```python
from build123d import *

# Parameters (mm, degrees)
F1_DEPTH = 2
F2_R     = 4.445875
F3_DEPTH = 6
F4_R     = 4.445875
F5_DEPTH = 3
F6_R     = 1.6
F7_DEPTH = 11.001


with BuildPart() as f1:
    # F0 (on Top) → F1 (new body)
    with BuildSketch(Plane.XY):
        Polygon((20, 9.5026303193), (0, 18.5309549122), (-20, 9.5026303193), (-20, -12.4407204949), (0, -21.4690450878), (20, -12.4407204949), align=None)
    extrude(amount=-F1_DEPTH)

    # F2 (on face) → F3 (join)
    with BuildSketch(Plane.XY):
        Circle(F2_R)
    extrude(amount=F3_DEPTH)

    # F4 (on face) → F5 (join)
    with BuildSketch(Plane(origin=(0, 0, -2), x_dir=(1, 0, 0), z_dir=(0, 0, -1))):
        Circle(F4_R)
    extrude(amount=F5_DEPTH)

    # F6 (on face) → F7 (cut, through all)
    with BuildSketch(Plane.XY.offset(6)):
        Circle(F6_R)
    extrude(amount=-F7_DEPTH, mode=Mode.SUBTRACT)


solid = f1.part
```
Geometry: final body of the model. Coordinates: model frame, mm. A direction names the side the tool comes from. Coordinates: 2 decimals unless noted, no trailing zeros. Order: outer loops, then holes, each group sorted by start corner. A loop starts at its lowest first (then second) coordinate and runs counter-clockwise, first axis right, second up. Notation, with made-up numbers: M 17,24.5 L 38,24.5 A26 cw 38,46.5 Z; hole C -33,28.5 d11. An arc over 180 degrees is marked long. Answer in a Markdown table with one row per item. Add a question column.
Q1. Contact query for flat-ended pins moving along their axis: P1, Ø2, axis at y = -5, z = 4.5, coming from the +X side; P2, Ø1, axis at x = -3.5, z = -1.5, coming from the -Y side; P3, Ø8, axis at x = 3.5, y = -16.5, coming from the +Z side. Output: stop coordinate, or through.
Q2. Mould query, pull axis Y, two halves, no side actions, for faces 1 (the cylindrical face through (-1.27, -0.97, 0.58)), 2 (the flat face through (-10.14, -16.89, -0.99)), 3 (the flat face through (0, -6, 0)). Classes: released by +Y, released by -Y, zero draft, split by the parting line, or undercut.
Q3. Section query A-A on y = 0. Return the cut outline in (x, z).
Q4. Section query C-C on y = -7. Return the cut outline in (x, z).
Q5. Line query: L1, parallel to Y at x = 0, z = -2.5; L2, parallel to Y at x = 0, z = -0.5; L3, parallel to Z at x = 5.5, y = -13. Output: solid intervals per line, ascending.
Q6. Reachability of faces 4 (the cylindrical face through (4.24, -1.34, -3.48)), 5 (the flat face through (20, -2, -1)), 6 (the cylindrical face through (4.24, 1.34, 2.96)) from +Z, -Z, +X, -X, +Y, -Y: full face, straight path, thin tool, end or side. Return the list, or none.
Q7. Section query B-B on z = 4.25. Return the cut outline in (x, y), and give its area (3 significant figures).
Q8. Section query D-D on x = 10. Return the cut outline in (y, z), and give its area (3 significant figures).
Completed:
| question | item | result |
|---|---|---|
| 1 | P1 | stops at x = 1.94 |
| 1 | P2 | stops at y = -20.11 |
| 1 | P3 | stops at z = 0 |
| 2 | face 1 | undercut |
| 2 | face 2 | released by -Y |
| 2 | face 3 | zero draft |
| 3 | outline | M -20,-2 L -4.45,-2 L -4.45,-5 L -1.6,-5 L -1.6,6 L -4.45,6 L -4.45,0 L -20,0 Z; M 1.6,-5 L 4.45,-5 L 4.45,-2 L 20,-2 L 20,0 L 4.45,0 L 4.45,6 L 1.6,6 Z |
| 4 | outline | M -20,-2 L 20,-2 L 20,0 L -20,0 Z |
| 5 | L1 | y = -4.45 to -1.6, 1.6 to 4.45 |
| 5 | L2 | y = -21.47 to -1.6, 1.6 to 18.53 |
| 5 | L3 | z = -2 to 0 |
| 6 | face 4 | -Z |
| 6 | face 5 | +Z, -Z, +X, +Y, -Y |
| 6 | face 6 | +Z |
| 7 | outline | C 0,0 d8.89; hole C 0,0 d3.2 |
| 7 | area | 54.1 mm2 |
| 8 | outline | M -16.95,-2 L 14.02,-2 L 14.02,0 L -16.95,0 Z |
| 8 | area | 61.9 mm2 |
